from build123d import *

# Parameters (mm, degrees)
ESQUISSE1_W             = 24
ESQUISSE1_H             = 25
BOSS_EXTRU_1_DEPTH      = 3
CONG_3_R                = 7.5
ENL_V_MAT_EXTRU_1_REACH = 36.785
ESQUISSE2_R             = 1.5
ENL_V_MAT_EXTRU_2_REACH = 36.785
ESQUISSE3_W             = 8
ESQUISSE3_H             = 3
ENL_V_MAT_EXTRU_3_REACH = 36.785
ESQUISSE4_W             = 5.5
ESQUISSE4_H             = 3
ENL_V_START             = -3
ESQUISSE5_W             = 3.5
ESQUISSE5_H             = 11
ENL_V_MAT_EXTRU_4_DEPTH = 3
ENL_V_MAT_EXTRU_5_REACH = 36.785
ENL_V_MAT_EXTRU_6_REACH = 36.785


with BuildPart() as part:
    # Esquisse1 → Boss.-Extru.1 (new body)
    with BuildSketch(Plane.XY):
        with Locations((12, 12.5)):
            Rectangle(ESQUISSE1_W, ESQUISSE1_H)
    extrude(amount=BOSS_EXTRU_1_DEPTH)

    # Congé3
    cong_3_edges = [part.edges().sort_by_distance(p)[0] for p in [
        (0, 25, 1.5),
        (24, 25, 1.5),
    ]]
    fillet(cong_3_edges, radius=CONG_3_R)

    # Esquisse2 → Enlèv. mat.-Extru.1 (cut, up to next)
    with BuildSketch(Plane.XY.offset(3), mode=Mode.PRIVATE) as enl_v_mat_extru_1_sk1:
        with Locations((12, 18)):
            Circle(ESQUISSE2_R)
    enl_v_mat_extru_1_tool1 = extrude(enl_v_mat_extru_1_sk1.sketch, amount=-ENL_V_MAT_EXTRU_1_REACH, mode=Mode.PRIVATE) & part.part
    add(enl_v_mat_extru_1_tool1.solids().sort_by_distance((12, 18, 3))[0], mode=Mode.SUBTRACT)

    # Esquisse3 → Enlèv. mat.-Extru.2 (cut, up to next)
    with BuildSketch(Plane.XY.offset(3), mode=Mode.PRIVATE) as enl_v_mat_extru_2_sk1:
        with Locations((12, 1.5)):
            Rectangle(ESQUISSE3_W, ESQUISSE3_H)
    enl_v_mat_extru_2_tool1 = extrude(enl_v_mat_extru_2_sk1.sketch, amount=-ENL_V_MAT_EXTRU_2_REACH, mode=Mode.PRIVATE) & part.part
    add(enl_v_mat_extru_2_tool1.solids().sort_by_distance((12, 1.5, 3))[0], mode=Mode.SUBTRACT)

    # Esquisse4 → Enlèv. mat.-Extru.3 (cut, up to next)
    with BuildSketch(Plane.XY.offset(3), mode=Mode.PRIVATE) as enl_v_mat_extru_3_sk1:
        with Locations((12, 7.5)):
            Rectangle(ESQUISSE4_W, ESQUISSE4_H)
    enl_v_mat_extru_3_tool1 = extrude(enl_v_mat_extru_3_sk1.sketch, amount=-ENL_V_MAT_EXTRU_3_REACH, mode=Mode.PRIVATE) & part.part
    add(enl_v_mat_extru_3_tool1.solids().sort_by_distance((12, 7.5, 3))[0], mode=Mode.SUBTRACT)

    # Esquisse5 → Enlèv. mat.-Extru.4 (cut)
    with BuildSketch(Plane.XY.offset(3).offset(ENL_V_START)):
        with Locations((12, 5.5)):
            Rectangle(ESQUISSE5_W, ESQUISSE5_H)
    extrude(amount=ENL_V_MAT_EXTRU_4_DEPTH, mode=Mode.SUBTRACT)

    # Esquisse6 → Enlèv. mat.-Extru.5 (cut, up to next)
    with BuildSketch(Plane.XY.offset(3), mode=Mode.PRIVATE) as enl_v_mat_extru_5_sk1:
        with BuildLine():
            Line((17.5, 14.25), (30.5, 14.25))
            ThreePointArc((30.5, 14.25), (31.25, 13.5), (30.5, 12.75))
            Line((30.5, 12.75), (17.5, 12.75))
            ThreePointArc((17.5, 12.75), (16.75, 13.5), (17.5, 14.25))
        make_face()
    enl_v_mat_extru_5_tool1 = extrude(enl_v_mat_extru_5_sk1.sketch, amount=-ENL_V_MAT_EXTRU_5_REACH, mode=Mode.PRIVATE) & part.part
    add(enl_v_mat_extru_5_tool1.solids().sort_by_distance((24, 13.5, 3))[0], mode=Mode.SUBTRACT)

    # Esquisse7 → Enlèv. mat.-Extru.6 (cut, up to next)
    with BuildSketch(Plane.XY.offset(3), mode=Mode.PRIVATE) as enl_v_mat_extru_6_sk1:
        with BuildLine():
            Line((-5.5, 14.25), (5.5, 14.25))
            ThreePointArc((5.5, 14.25), (6.25, 13.5), (5.5, 12.75))
            Line((5.5, 12.75), (-5.5, 12.75))
            ThreePointArc((-5.5, 12.75), (-6.25, 13.5), (-5.5, 14.25))
        make_face()
    enl_v_mat_extru_6_tool1 = extrude(enl_v_mat_extru_6_sk1.sketch, amount=-ENL_V_MAT_EXTRU_6_REACH, mode=Mode.PRIVATE) & part.part
    add(enl_v_mat_extru_6_tool1.solids().sort_by_distance((0, 13.5, 3))[0], mode=Mode.SUBTRACT)


solid = part.part
Source: CAD feature listing. Evaluate the final solid. Frame: model axes, mm. A direction names the side the tool comes from. Round coordinates to 2 decimals unless told otherwise and drop trailing zeros. Loops run counter-clockwise (first coordinate to the right, second up) from the corner with the lowest first, then second, coordinate; pieces in that order, holes last.
Q1. Mould query, pull axis X, two halves, no side actions, for faces 1 (the face through (4, 0, 1)), 2 (the face through (9.25, 7, 2)), 3 (the face through (6.25, 13.52, 1.52)). Classes: pulls with the +X half, pulls with the -X half, needs draft (parallel to the pull), parting line crosses it, or undercut.
Q2. Section C-C, the plane y = 18.5. Return loops of the section in (x, z), plus the area to 3 significant figures.
Q3. First-contact query: P1, Ø1.5, axis at y = 7.5, z = 1, coming from the -X side; P2, Ø1.1, axis at x = 10, z = 1.5, coming from the -Y side; P3, Ø0.9, axis at x = 12.5, z = 1, coming from the -Y side. Flat tips, straight axial feed; report the tip coordinate or a pass-through.
Q4. Section A-A, the plane x = 22.5. Return loops of the section in (y, z), plus the area to 3 significant figures.
Q5. Ray query, line 1 (X direction, y = 8.5, z = 1.25); line 2 (Y direction, x = 12, z = 1); line 3 (X direction, y = 10, z = 2.9). Return the intervals inside material, ascending.
Q6. Section D-D, the plane y = 13.5. Return loops of the section in (x, z), plus the area to 3 significant figures.
Q7. Access query for faces 4 (the face through (10, 9, 2)), 5 (the face through (13.75, 4, 1)), 6 (the face through (21, 12.75, 2)), 7 (the face through (3, 12.75, 2)). Directions: +Z, -Z, +X, -X, +Y, -Y. A direction counts if a zero-diameter tool reaches every point of the face in a straight line with its end or side. Return the directions, or none.
Solutions:
1. face 1: needs draft
1. face 2: undercut
1. face 3: pulls with the -X half
2. outline: (0.07, 0) - (10.59, 0) - (10.59, 3) - (0.07, 3) - close; (13.41, 0) - (23.93, 0) - (23.93, 3) - (13.41, 3) - close
2. area: 63.1 mm2
3. P1: stops at x = 0
3. P2: stops at y = 3
3. P3: stops at y = 11
4. outline: (0, 0) - (12.75, 0) - (12.75, 3) - (0, 3) - close; (14.25, 0) - (22, 0) - (22, 3) - (14.25, 3) - close
4. area: 61.5 mm2
5. line 1: x = 0 to 9.25, 14.75 to 24
5. line 2: y = 11 to 16.5, 19.5 to 25
5. line 3: x = 0 to 10.25, 13.75 to 24
6. outline: (6.25, 0) - (16.75, 0) - (16.75, 3) - (6.25, 3) - close
6. area: 31.5 mm2
7. face 4: +Z, -Z
7. face 5: +Z, -Z, -Y
7. face 6: +Z, -Z, +X
7. face 7: +Z, -Z, -X
